from build123d import *

# Parameters (mm, degrees)
SKETCH_1_R      = 1.6
SKETCH_1_R_2    = 3.5
SKETCH_1_R_3    = 25
SKETCH_1_R_4    = 10
EXTRUDE_1_DEPTH = 5


with BuildPart() as part:
    # 草图1 → 凸台-拉伸1 (new body)
    # profile 1 of 4: a face of its own
    with BuildSketch(Plane(origin=(0, 0, 0), x_dir=(1, 0, 0), z_dir=(0, 1, 0))):
        with BuildLine():
            ThreePointArc((25, 56.96), (0, 31.96), (-25, 56.96))
            Line((-25, 56.96), (-25, -56.96))
            ThreePointArc((-25, -56.96), (0, -31.96), (25, -56.96))
            ThreePointArc((25, -56.96), (23.096988313, -66.527085809), (17.67766953, -74.63766953))
            Line((17.67766953, -74.63766953), (74.63766953, -17.67766953))
            ThreePointArc((74.63766953, -17.67766953), (31.96, 0), (74.63766953, 17.67766953))
            Line((74.63766953, 17.67766953), (17.67766953, 74.63766953))
            ThreePointArc((17.67766953, 74.63766953), (23.096988313, 66.527085809), (25, 56.96))
        make_face()
        with Locations(Location((0, -7, 0), (0, 0, 270))):
            Circle(SKETCH_1_R, mode=Mode.SUBTRACT)
        with Locations(Location((-7, 0, 0), (0, 0, 270))):
            Circle(SKETCH_1_R, mode=Mode.SUBTRACT)
        with Locations(Location((0, 0, 0), (0, 0, 270))):
            Circle(SKETCH_1_R_2, mode=Mode.SUBTRACT)
        with Locations(Location((0, 7, 0), (0, 0, 270))):
            Circle(SKETCH_1_R, mode=Mode.SUBTRACT)
        with Locations(Location((7, 0, 0), (0, 0, 270))):
            Circle(SKETCH_1_R, mode=Mode.SUBTRACT)
    # profile 2 of 4: a face of its own
    with BuildSketch(Plane(origin=(0, 0, 0), x_dir=(1, 0, 0), z_dir=(0, 1, 0))):
        with Locations((0, -56.96)):
            Circle(SKETCH_1_R_3)
        with Locations(Location((0, -56.96, 0), (0, 0, 270))):
            Circle(SKETCH_1_R_4, mode=Mode.SUBTRACT)
    # profile 3 of 4: a face of its own
    with BuildSketch(Plane(origin=(0, 0, 0), x_dir=(1, 0, 0), z_dir=(0, 1, 0))):
        with Locations((56.96, 0)):
            Circle(SKETCH_1_R_3)
        with Locations(Location((56.96, 0, 0), (0, 0, 270))):
            Circle(SKETCH_1_R_4, mode=Mode.SUBTRACT)
    # profile 4 of 4: a face of its own
    with BuildSketch(Plane(origin=(0, 0, 0), x_dir=(1, 0, 0), z_dir=(0, 1, 0))):
        with Locations((0, 56.96)):
            Circle(SKETCH_1_R_3)
        with Locations(Location((0, 56.96, 0), (0, 0, 270))):
            Circle(SKETCH_1_R_4, mode=Mode.SUBTRACT)
    extrude(amount=EXTRUDE_1_DEPTH)


solid = part.part
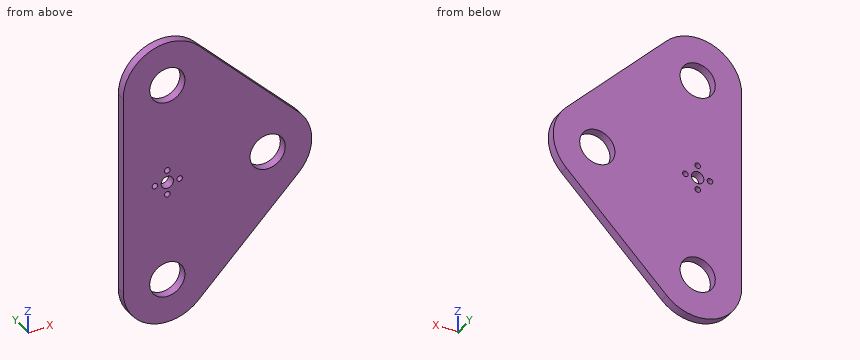
Input: part model. Units: mm. Frame: model coordinates. Coordinates: 2 decimals unless noted, no trailing zeros. Order: outer loops, then holes, each group sorted by start corner. A loop starts at its lowest first (then second) coordinate and runs counter-clockwise, first axis right, second up. Notation, with made-up numbers: M -29,17 L -21,17 A9 cw -21,26 Z; hole C 10,1.25 d3. An arc over 180 degrees is marked long. Write item = value, one per line. Start each with the question number.
(1) Section C-C on y = 1.6. Give the number of separate pieces and of enclosed holes in the cut face, and give its area (3 significant figures).
(2) Line query: line 1 along X through (y, z) = (2.15, 0); line 2 along Z through (x, y) = (-7.5, 3); line 3 along X through (y, z) = (2.75, 1). Output: solid intervals per line, ascending. Write a range as [from, to].
(3) Section D-D on z = 51. Output: boundary loops of the cut face in (x, y), and give its area (3 significant figures).
(4) First-contact query: P1, Ø1, axis at x = 46, y = 4, coming from the -Z side; P2, Ø18, axis at x = 56.96, z = 0, coming from the +Y side; P3, Ø3, axis at y = 3.5, z = 8, coming from the +X side; P4, Ø1, axis at y = 2.5, z = 6, coming from the +X side. Flat tips, straight axial feed; report the tip coordinate or a pass-through.
(5) Section A-A on z = 0. Output: boundary loops of the cut face in (x, y), and give its area (3 significant figures).
(6) Section B-B on x = -7. Output: boundary loops of the cut face in (y, z).
Result set:
q1.separate_pieces = 1
q1.enclosed_holes = 8
q1.area = 11,100 mm²
q2.line_1 = [-25, -8.6], [-5.4, -3.5], [3.5, 5.4], [8.6, 46.96], [66.96, 81.96]
q2.line_2 = [-80.81, -63.57], [-50.35, -1.52], [1.52, 50.35], [63.57, 80.81]
q2.line_3 = [-25, -8.25], [-5.75, -3.35], [3.35, 5.75], [8.25, 47.01], [66.91, 81.94]
q3.outline = M -25,0 L -8.03,0 L -8.03,5 L -25,5 Z; M 8.03,0 L 41.32,0 L 41.32,5 L 8.03,5 Z
q3.area = 251 mm²
q4.P1 = -46.82
q4.P2 = through
q4.P3 = 81.1
q4.P4 = 81.35
q5.outline = M -25,0 L -8.6,0 L -8.6,5 L -25,5 Z; M -5.4,0 L -3.5,0 L -3.5,5 L -5.4,5 Z; M 3.5,0 L 5.4,0 L 5.4,5 L 3.5,5 Z; M 8.6,0 L 46.96,0 L 46.96,5 L 8.6,5 Z; M 66.96,0 L 81.96,0 L 81.96,5 L 66.96,5 Z
q5.area = 368 mm²
q6.outline = M 0,-80.96 L 5,-80.96 L 5,-64.1 L 0,-64.1 Z; M 0,-49.82 L 5,-49.82 L 5,-1.6 L 0,-1.6 Z; M 0,1.6 L 5,1.6 L 5,49.82 L 0,49.82 Z; M 0,64.1 L 5,64.1 L 5,80.96 L 0,80.96 Z
